Verification items for the finished model (mm, model axes). A direction names the side the tool comes from. Round coordinates to 2 decimals unless told otherwise and drop trailing zeros. Loops run counter-clockwise (first coordinate to the right, second up) from the corner with the lowest first, then second, coordinate; pieces in that order, holes last. Notation, with made-up numbers: M 84,27.25 L 109,27.25 A14 ccw 109,36.25 Z; hole C 64,-32.5 d4. An arc over 180 degrees is marked long. One line per item, written item: value.
from build123d import *

# Parameters (mm, degrees)
BOSS_EXTRUDE1_DEPTH = 20


with BuildPart() as part:
    # Sketch1 → Boss-Extrude1 (new body)
    with BuildSketch(Plane(origin=(0, 0, 0), x_dir=(1, 0, 0), z_dir=(0, 1, 0))):
        with BuildLine():
            Line((-2.966479395, 0.9), (-4, 0.9))
            Line((-4, 0.9), (-4, -0.9))
            Line((-4, -0.9), (-2.966479395, -0.9))
            ThreePointArc((-2.966479395, -0.9), (-3.1, 0), (-2.966479395, 0.9))
        make_face()
        with BuildLine():
            Line((4, 0.9), (2.966479395, 0.9))
            ThreePointArc((2.966479395, 0.9), (3.066438172, 0.4549252), (3.1, 0))
            ThreePointArc((3.1, 0), (3.066438172, -0.4549252), (2.966479395, -0.9))
            Line((2.966479395, -0.9), (4, -0.9))
            Line((4, -0.9), (4, 0.9))
        make_face()
        with BuildLine():
            Line((2.966479395, 0.9), (-2.966479395, 0.9))
            ThreePointArc((-2.966479395, 0.9), (-3.1, 0), (-2.966479395, -0.9))
            Line((-2.966479395, -0.9), (2.966479395, -0.9))
            ThreePointArc((2.966479395, -0.9), (3.066438172, -0.4549252), (3.1, 0))
            ThreePointArc((3.1, 0), (3.066438172, 0.4549252), (2.966479395, 0.9))
        make_face()
        with BuildLine():
            Line((2.966479395, -0.9), (-2.966479395, -0.9))
            ThreePointArc((-2.966479395, -0.9), (0, -3.1), (2.966479395, -0.9))
        make_face()
        with BuildLine():
            ThreePointArc((2.966479395, 0.9), (0, 3.1), (-2.966479395, 0.9))
            Line((-2.966479395, 0.9), (2.966479395, 0.9))
        make_face()
    extrude(amount=BOSS_EXTRUDE1_DEPTH)


solid = part.part
(1) Thickness scan on L1, parallel to Z at x = 3, y = 14.5; L2, parallel to X at y = 2.5, z = 1.5; L3, parallel to X at y = 8.75, z = -2.5. Record the ranges inside material, lowest first. Write a range as from..to.
Completed:
L1: z = -0.9..0.9
L2: x = -2.71..2.71
L3: x = -1.83..1.83
(2) Sectioned sample at B-B on z = 2.25. Enter the section's corners in (x, y), and give its area (3 significant figures).
Completed:
outline: M -2.13,0 L 2.13,0 L 2.13,20 L -2.13,20 Z
area: 85.3 mm^2
(3) Sectioned sample at A-A on y = 3.5. Enter the section's corners in (x, z), and give its area (3 significant figures).
Completed:
outline: M -4,-0.9 L -2.97,-0.9 A3.1 ccw 2.97,-0.9 L 4,-0.9 L 4,0.9 L 2.97,0.9 A3.1 ccw -2.97,0.9 L -4,0.9 Z
area: 33.6 mm^2
(4) Sectioned sample at C-C on x = -1.5. Enter the section's corners in (y, z), and give its area (3 significant figures).
Completed:
outline: M 0,-2.71 L 20,-2.71 L 20,2.71 L 0,2.71 Z
area: 109 mm^2
(5) Tool access check on faces 1 (the face through (-3.5, 9.9, 0.9)), 2 (the face through (3.5, 9.9, 0.9)), 3 (the face through (3.5, 9.9, -0.9)), 4 (the face through (-3.5, 9.9, -0.9)). Record the directions out of +Z, -Z, +X, -X, +Y, -Y that give a thin tool (end or side, any length) a straight path to the whole face; none if there is none.
Completed:
face 1: +Z, -X, +Y, -Y
face 2: +Z, +X, +Y, -Y
face 3: -Z, +X, +Y, -Y
face 4: -Z, -X, +Y, -Y
(6) Depth check by flat-ended pin: pin 1 Ø0.8 at (x, y) = (-3.5, 14) entering from -Z; pin 2 Ø0.5 at (x, y) = (3.5, 9) entering from +Z; pin 3 Ø1 at (x, y) = (-3, 16) entering from -Z. Enter the tip coordinate at first touch or a pass-through.
Completed:
pin 1: stops at z = -0.9
pin 2: stops at z = 0.9
pin 3: stops at z = -1.83
